```python
from build123d import *

# Parameters (mm, degrees)
BOSS_EXTRU_1_DEPTH      = 8.9916
ESQUISSE2_R             = 9.906
BOSS_EXTRU_2_DEPTH      = 12.7
BOSS_EXTRU_3_DEPTH      = 6.096
CONG_1_R                = 2.54
ESQUISSE4_W             = 28.956
ESQUISSE4_H             = 9.017
BOSS_EXTRU_4_DEPTH      = 9.2202
ESQUISSE5_W             = 39.751
ESQUISSE5_H             = 17.78
BOSS_EXTRU_5_DEPTH      = 40.132
ESQUISSE6_R             = 4.4069
BOSS_EXTRU_6_DEPTH      = 39.751
ESQUISSE7_R             = 2.921
ENL_V_MAT_EXTRU_1_DEPTH = 2.54
ESQUISSE8_R             = 1.825
BOSS_EXTRU_7_DEPTH      = 50.8


with BuildPart() as part:
    # Esquisse1 → Boss.-Extru.1 (new, symmetric)
    with BuildSketch(Plane(origin=(0, 0, 0), x_dir=(1, 0, 0), z_dir=(0, 1, 0))):
        with BuildLine():
            Line((-23.8379, 15.9766), (23.8379, 15.9766))
            ThreePointArc((23.8379, 15.9766), (39.8145, 0), (23.8379, -15.9766))
            Line((23.8379, -15.9766), (-23.8379, -15.9766))
            ThreePointArc((-23.8379, -15.9766), (-39.8145, 0), (-23.8379, 15.9766))
        make_face()
    extrude(amount=BOSS_EXTRU_1_DEPTH, both=True)

    # Esquisse2 → Boss.-Extru.2 (add)
    with BuildSketch(Plane(origin=(0, 8.9916, 0), x_dir=(1, 0, 0), z_dir=(0, 1, 0))):
        with Locations(Location((0, 0, 0), (0, 0, 270))):
            Circle(ESQUISSE2_R)
    extrude(amount=BOSS_EXTRU_2_DEPTH)

    # Esquisse3 → Boss.-Extru.3 (add)
    with BuildSketch(Plane.XZ.offset(8.9916)):
        with BuildLine():
            Line((-10.795, 9.525), (10.795, 9.525))
            ThreePointArc((10.795, 9.525), (20.32, 0), (10.795, -9.525))
            Line((10.795, -9.525), (-10.795, -9.525))
            ThreePointArc((-10.795, -9.525), (-20.32, 0), (-10.795, 9.525))
        make_face()
    extrude(amount=BOSS_EXTRU_3_DEPTH)

    # Congé1
    cong_1_edges = [part.edges().sort_by_distance(p)[0] for p in [
        (-20.32, -8.9916, 0),
        (0, -8.9916, -9.525),
        (20.32, -8.9916, 0),
        (0, -8.9916, 9.525),
    ]]
    fillet(cong_1_edges, radius=CONG_1_R)

    # Esquisse4 → Boss.-Extru.4 (add)
    with BuildSketch(Plane.XZ.offset(15.0876)):
        Rectangle(ESQUISSE4_W, ESQUISSE4_H)
    extrude(amount=BOSS_EXTRU_4_DEPTH)

    # Esquisse5 → Boss.-Extru.5 (add)
    with BuildSketch(Plane.XZ.offset(24.3078)):
        Rectangle(ESQUISSE5_W, ESQUISSE5_H)
    extrude(amount=BOSS_EXTRU_5_DEPTH)

    # Esquisse6 → Boss.-Extru.6 (add)
    with BuildSketch(Plane(origin=(19.8755, 0, 0), x_dir=(0, 0, -1), z_dir=(1, 0, 0))):
        with Locations((0, -64.4398)):
            Circle(ESQUISSE6_R)
    extrude(amount=-BOSS_EXTRU_6_DEPTH)

    # Esquisse7 → Enlèv. mat.-Extru.1 (cut)
    with BuildSketch(Plane(origin=(0, 0, -8.89), x_dir=(-1, 0, 0), z_dir=(0, 0, -1))):
        with Locations((0, -45.487412675)):
            Circle(ESQUISSE7_R)
    extrude(amount=-ENL_V_MAT_EXTRU_1_DEPTH, mode=Mode.SUBTRACT)

    # Esquisse8 → Boss.-Extru.7 (add)
    with BuildSketch(Plane.XZ.offset(8.9916)):
        with Locations(Location((26.513063704, 8.491811342, 0), (0, 0, 90))):
            Circle(ESQUISSE8_R)
    extrude(amount=BOSS_EXTRU_7_DEPTH)


solid = part.part
```
Can you work these out from the model? Positions are in its coordinate system, mm. A direction names the side the tool comes from. Coordinates: 2 decimals unless noted, no trailing zeros. Loops run counter-clockwise (first coordinate to the right, second up) from the corner with the lowest first, then second, coordinate; pieces in that order, holes last.
1) Imagine slicing it at D-D on y = 5. List the corners of the cut face in (x, z) for me, plus the area to 3 significant figures.
2) Imagine slicing it at B-B on z = 0. List the corners of the cut face in (x, y) for me.
3) Thinking about a two-plate mould opening in Y: for faces 6 (the flat face through (0, -20, -4.508)), 7 (the flat face through (0, 21.692, 0)), 8 (the flat face through (4, -44, -8.89)), 9 (the cylindrical face through (0.151, -9.716, 10.289)), which applies, pulls with the +Y half, pulls with the -Y half, needs draft (parallel to the pull), parting line crosses it, or undercut?
4) I need wall thicknesses on probe 1 along Y at (x, z) = (0, -7); probe 2 along Z at (x, y) = (19, -44.5); probe 3 along Y at (x, z) = (-28.5, 10). Which ranges of each line are inside material? Lowest first, please.
5) For pin 1 (4.5 mm diameter, centred on x = -7, y = -19.5, fed in from +Z); pin 2 (2 mm diameter, centred on x = 2.5, z = -7.5, fed in from -Y); pin 3 (1.1 mm diameter, centred on x = 0, y = -13, fed in from -Z) (3 decimals), each with a flat end and sliding along its axis, tell me the tip position at first contact or that it passes through.
6) Which directions (+Z, -Z, +X, -X, +Y, -Y) give clear straight access to the entire face, cutting with the end or side of a thin tool? Please do faces 1 (the flat face through (0, -20, 4.508)), 2 (the flat face through (-14.478, -20, 0)), 3 (the flat face through (0, -64.44, -7)), 4 (the cylindrical face through (20.318, -13.285, 0.209)), 5 (the flat face through (14.478, -20, 0)).
Completed:
1. outline: (-23.84, -15.98) - (23.84, -15.98) arc R15.98 ccw to (23.84, 15.98) - (-23.84, 15.98) arc R15.98 ccw to start
1. area: 2,330 mm2
2. outline: (-39.81, -8.99) - (-22.86, -8.99) arc R2.54 cw to (-20.32, -11.53) - (-20.32, -15.09) - (-14.48, -15.09) - (-14.48, -24.31) - (-19.88, -24.31) - (-19.88, -68.85) - (19.88, -68.85) - (19.88, -24.31) - (14.48, -24.31) - (14.48, -15.09) - (20.32, -15.09) - (20.32, -11.53) arc R2.54 cw to (22.86, -8.99) - (39.81, -8.99) - (39.81, 8.99) - (9.91, 8.99) - (9.91, 21.69) - (-9.91, 21.69) - (-9.91, 8.99) - (-39.81, 8.99) - close
3. face 6: undercut
3. face 7: pulls with the +Y half
3. face 8: needs draft
3. face 9: pulls with the -Y half
4. probe 1: y = -64.44 to -48.41, -42.57 to -24.31, -15.09 to 21.69
4. probe 2: z = -8.89 to 8.89
4. probe 3: y = -8.99 to 8.99
5. pin 1: stops at z = 4.51
5. pin 2: stops at y = -64.44
5. pin 3: stops at z = -9.525
6. face 1: +Z, +X, -X
6. face 2: +Z, -Z, -X
6. face 3: -Z, +X, -X, -Y
6. face 4: none
6. face 5: +Z, -Z, +X
